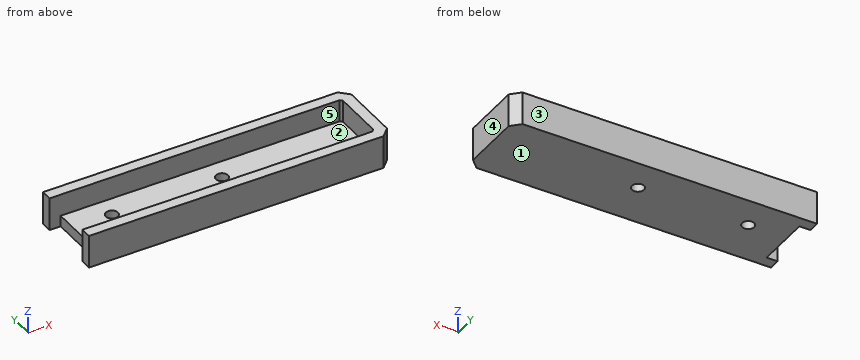
from build123d import *

# Parameters (mm, degrees)
SKETCH1_R           = 2.75
BOSS_EXTRUDE1_DEPTH = 5
BOSS_EXTRUDE4_DEPTH = 15


with BuildPart() as part:
    # Sketch1 → Boss-Extrude1 (new body)
    with BuildSketch(Plane.XY):
        Polygon((72.390908062, 0), (72.390908062, -25), (195, -25), (199, -25), (200, -24), (200, -1), (199, 0), (195, 0), align=None)
        with Locations(Location((90, -9.5, 0), (0, 0, 180))):
            Circle(SKETCH1_R, mode=Mode.SUBTRACT)
        with Locations(Location((140, -9.5, 0), (0, 0, 180))):
            Circle(SKETCH1_R, mode=Mode.SUBTRACT)
    extrude(amount=BOSS_EXTRUDE1_DEPTH)

    # Sketch2 → Boss-Extrude4 (add)
    with BuildSketch(Plane(origin=(0, 0, 0), x_dir=(-1, 0, 0), z_dir=(0, 0, -1))):
        Polygon((-72.390908062, 0), (-199, 0), (-200, -1), (-200, -24), (-199, -25), (-72.390908062, -25), (-67.390908062, -25), (-67.390908062, -30), (-201.071067812, -30), (-205, -26.071067812), (-205, 1.071067812), (-201.071067812, 5), (-67.390908062, 5), (-67.390908062, 0), align=None)
    extrude(amount=-BOSS_EXTRUDE4_DEPTH)


solid = part.part
CAD build for the part. Positions are in the model's coordinates, mm. Face numbers are marked on the shaded views. A direction names the side the tool comes from. Coordinates: 2 decimals unless noted, no trailing zeros. Write each loop counter-clockwise with the first axis right and the second up, starting at its lowest first coordinate (ties: lowest second). Pieces come first, ordered by that corner, then holes. Notation, with made-up numbers: (14.25, -23.5) - (34.25, -23.5) arc R15 ccw to (34.25, 1.5) - close; hole circle Ø3 at (85.25, 45.25). An arc over 180 degrees is marked (long way). Use a Markdown table: item, result. Add a question column.
Item 1: Flat gauge pins, fed straight in: pin 1 (1.5 mm diameter, centred on y = -9.5, z = 2.5, fed in from -X); pin 2 (3 mm diameter, centred on y = -12.5, z = 9, fed in from -X); pin 3 (2 mm diameter, centred on x = 159.5, y = -8, fed in from +Z); pin 4 (3.5 mm diameter, centred on x = 140, y = -9.5, fed in from +Z). Where does each tip first touch, or does it go through?
Item 2: Drill centre lines: L1, parallel to X at y = -9.5, z = 2.5; L2, parallel to Y at x = 140, z = 1.8; L3, parallel to Y at x = 160, z = 13. Where is each one in solid material? Low to high. Write a range as from..to.
Item 3: Band-saw the part on B-B, the plane x = 90. Give the cut face in (y, z).
Item 4: Band-saw the part on D-D, the plane z = 11.25. Give the cut face in (x, y).
Item 5: Band-saw the part on A-A, the plane y = -9.5. Give the cut face in (x, z), and give its area (3 significant figures).
Item 6: Band-saw the part on C-C, the plane z = 1.5. Give the cut face in (x, y), and give its area (3 significant figures).
Item 7: 3-axis set-ups, long thin cutter, end or side, ignore diameter. For the marked faces 4 and 5: which of +Z, -Z, +X, -X, +Y, -Y reach the whole face in a straight line?
Item 8: Mould opens along Y. For the marked faces 1, 2 and 3 say: pulls with the +Y half, pulls with the -Y half, needs draft (parallel to the pull), parting line crosses it, or undercut.
Numbers:
| question | item | result |
|---|---|---|
| 1 | pin 1 | x = 72.39 |
| 1 | pin 2 | x = 200 |
| 1 | pin 3 | z = 5 |
| 1 | pin 4 | through |
| 2 | L1 | 72.39..87.25, 92.75..137.25, 142.75..205 |
| 2 | L2 | -30..-12.25, -6.75..5 |
| 2 | L3 | -30..-25, 0..5 |
| 3 | outline | (-30, 0) - (-12.25, 0) - (-12.25, 5) - (-25, 5) - (-25, 15) - (-30, 15) - close; (-6.75, 0) - (5, 0) - (5, 15) - (0, 15) - (0, 5) - (-6.75, 5) - close |
| 4 | outline | (67.39, -30) - (201.07, -30) - (205, -26.07) - (205, 1.07) - (201.07, 5) - (67.39, 5) - (67.39, 0) - (199, 0) - (200, -1) - (200, -24) - (199, -25) - (67.39, -25) - close |
| 5 | outline | (72.39, 0) - (87.25, 0) - (87.25, 5) - (72.39, 5) - close; (92.75, 0) - (137.25, 0) - (137.25, 5) - (92.75, 5) - close; (142.75, 0) - (205, 0) - (205, 15) - (200, 15) - (200, 5) - (142.75, 5) - close |
| 5 | area | 658 mm2 |
| 6 | outline | (67.39, -30) - (201.07, -30) - (205, -26.07) - (205, 1.07) - (201.07, 5) - (67.39, 5) - (67.39, 0) - (72.39, 0) - (72.39, -25) - (67.39, -25) - close; hole circle Ø5.5 at (90, -9.5); hole circle Ø5.5 at (140, -9.5) |
| 6 | area | 4,630 mm2 |
| 7 | face 4 | +Z, -Z, +X, +Y, -Y |
| 7 | face 5 | +Z, -X |
| 8 | face 1 | needs draft |
| 8 | face 2 | undercut |
| 8 | face 3 | pulls with the +Y half |
